Check sheet for the drawn part. Datum: minimum x, y, z corner. Units: mm. A direction names the side the tool comes from. Coordinates: 2 decimals unless noted, no trailing zeros. Loops run counter-clockwise (first coordinate to the right, second up) from the corner with the lowest first, then second, coordinate; pieces in that order, holes last.
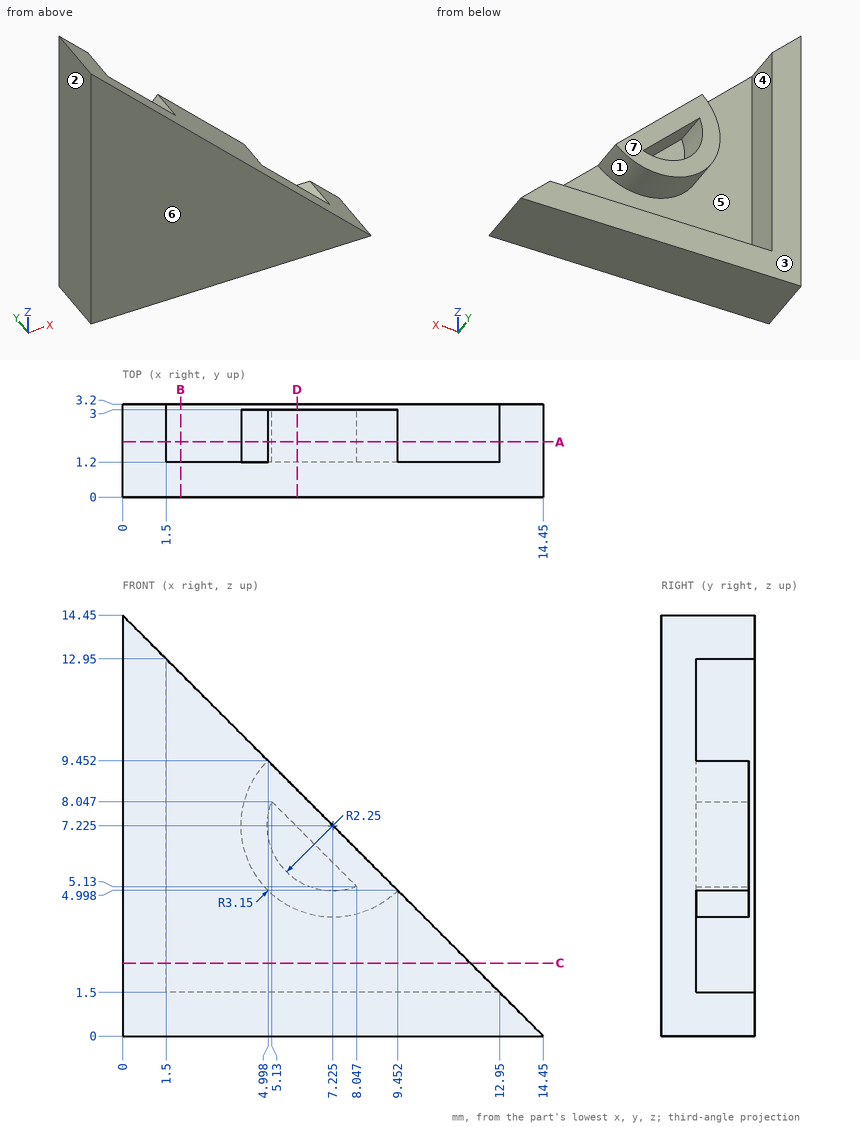
1) Depth check by flat-ended pin: pin 1 (2.5 mm diameter, centred on x = 7, z = 5.5, fed in from +Y); pin 2 (1.5 mm diameter, centred on y = 1.5, z = 8.5, fed in from +X); pin 3 (1 mm diameter, centred on x = 7.5, y = 2, fed in from +Z). Enter the tip coordinate at first touch or a pass-through.
Answer sheet:
pin 1: stops at y = 3
pin 2: stops at x = 6.7
pin 3: stops at z = 7.45
2) Section check B-B on x = 2. Enter the section's corners in (y, z).
Answer sheet:
outline: (0, 0) - (3.2, 0) - (3.2, 1.5) - (1.2, 1.5) - (1.2, 12.45) - (0, 12.45) - close
3) Section check D-D on x = 6. Enter the section's corners in (y, z).
Answer sheet:
outline: (0, 0) - (3.2, 0) - (3.2, 1.5) - (1.2, 1.5) - (1.2, 4.32) - (3, 4.32) - (3, 5.34) - (1.2, 5.34) - (1.2, 7.18) - (3, 7.18) - (3, 8.45) - (0, 8.45) - close
4) Section check C-C on z = 2.5. Enter the section's corners in (x, y).
Answer sheet:
outline: (0, 0) - (11.95, 0) - (11.95, 1.2) - (1.5, 1.2) - (1.5, 3.2) - (0, 3.2) - close
5) Set-up check for the marked faces 4, 5, 6 and 7: record each of +Z, -Z, +X, -X, +Y, -Y from which the full face is reachable in a straight line by a thin tool's end or side.
Answer sheet:
face 4: +Z, +Y
face 5: +Y
face 6: +Z, -Z, +X, -X, -Y
face 7: +Z, +X, +Y
6) Mould release check, pull along X, two halves, no side actions. Record for the marked faces 1, 2 and 3: +X half, -X half, draft (parallel to the pull), parting line (faces both ways), or undercut.
Answer sheet:
face 1: undercut
face 2: -X half
face 3: draft
7) Scan lines: line 1 (Z direction, x = 5.75, y = 2.8) (1 decimal); line 2 (Z direction, x = 6.75, y = 2.95) (1 decimal); line 3 (X direction, y = 2.4, z = 10.75). Record each from-to range of solid material in increasing order.
Answer sheet:
line 1: z = 0 to 1.5, 4.4 to 5.5, 7.4 to 8.7
line 2: z = 0 to 1.5, 4.1 to 5, 6.4 to 7.7
line 3: x = 0 to 1.5
8) Section check A-A on y = 1.9. Give the number of separate pieces and of enclosed holes in the cut face.
Answer sheet:
separate pieces: 2
enclosed holes: 1
